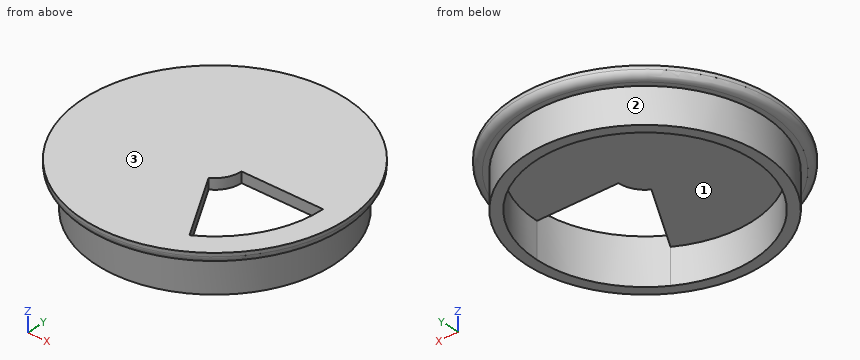
```python
from build123d import *

# Parameters (mm, degrees)
F0_R     = 37
F1_DEPTH = 3
F2_R     = 2
F3_R     = 33.5
F4_DEPTH = 10


with BuildPart() as f1:
    # F0 (on Top) → F1 (new body)
    with BuildSketch(Plane.XY):
        Circle(F0_R)
        with BuildLine():
            ThreePointArc((16.75, -29.0118510268), (-29.0118510268, 16.75), (33.5, 0))
            ThreePointArc((33.5, 0), (29.0118510268, -16.75), (16.75, -29.0118510268))
        make_face(mode=Mode.SUBTRACT)
        with BuildLine():
            Line((7.5, 0), (30.5, 0))
            ThreePointArc((30.5, 0), (-26.4137748154, 15.25), (15.25, -26.4137748154))
            Line((15.25, -26.4137748154), (3.75, -6.4951905284))
            ThreePointArc((3.75, -6.4951905284), (-6.4951905284, 3.75), (7.5, 0))
        make_face()
        with BuildLine():
            Line((30.5, 0), (33.5, 0))
            ThreePointArc((33.5, 0), (-29.0118510268, 16.75), (16.75, -29.0118510268))
            Line((16.75, -29.0118510268), (15.25, -26.4137748154))
            ThreePointArc((15.25, -26.4137748154), (-26.4137748154, 15.25), (30.5, 0))
        make_face()
        with BuildLine():
            ThreePointArc((3.75, -6.4951905284), (6.4951905284, -3.75), (7.5, 0))
            ThreePointArc((7.5, 0), (-6.4951905284, 3.75), (3.75, -6.4951905284))
        make_face()
        with BuildLine():
            ThreePointArc((16.75, -29.0118510268), (29.0118510268, -16.75), (33.5, 0))
            Line((33.5, 0), (30.5, 0))
            ThreePointArc((30.5, 0), (26.4137748154, -15.25), (15.25, -26.4137748154))
            Line((15.25, -26.4137748154), (16.75, -29.0118510268))
        make_face()
    extrude(amount=-F1_DEPTH)

    # F2
    f2_edges = [f1.edges().sort_by_distance(p)[0] for p in [
        (-37, 0, -3),
    ]]
    fillet(f2_edges, radius=F2_R)

    # F3 (on face) → F4 (join)
    with BuildSketch(Plane(origin=(0, 0, -3), x_dir=(1, 0, 0), z_dir=(0, 0, -1))):
        Circle(F3_R)
        with BuildLine():
            ThreePointArc((15.25, 26.4137748154), (26.4137748154, 15.25), (30.5, 0))
            ThreePointArc((30.5, 0), (-26.4137748154, -15.25), (15.25, 26.4137748154))
        make_face(mode=Mode.SUBTRACT)
    extrude(amount=F4_DEPTH)


solid = f1.part
```
Read the model definition and answer for the solid it produces. Units are mm, in the model's axes. Face numbers are marked on the shaded views. Coordinates: 2 decimals unless noted, no trailing zeros. Write each loop counter-clockwise with the first axis right and the second up, starting at its lowest first coordinate (ties: lowest second). Pieces come first, ordered by that corner, then holes. Notation, with made-up numbers: (75.25, -28) -> (112.25, -28) arc R35 cw to (112.25, 11) -> close; hole circle Ø2 at (-13, -18). An arc over 180 degrees is marked (long way). Return JSON: item names as keys, results as strings.
1. Each of these flat-tipped pins is pushed along its axis until it touches: P1, Ø1, axis at x = 13, z = -5.5, coming from the +Y side; P2, Ø6, axis at y = 18.5, z = -2.5, coming from the +X side; P3, Ø1, axis at x = -8.5, y = -15.5, coming from the +Z side; P4, Ø3.5, axis at x = 16, z = -2, coming from the -Y side. Where does it stop, or does it pass through?
Found:
{"P1": "y = 31.08", "P2": "x = 33.46", "P3": "z = 0", "P4": "y = -34.06"}
2. A cutting plane is placed at A-A (x = 0). Determine the outline of the cut face in (y, z).
Found:
{"outline": "(-37, -1) arc R2 ccw to (-35, -3) -> (-33.5, -3) -> (-33.5, -13) -> (-30.5, -13) -> (-30.5, -3) -> (30.5, -3) -> (30.5, -13) -> (33.5, -13) -> (33.5, -3) -> (35, -3) arc R2 ccw to (37, -1) -> (37, 0) -> (-37, 0) -> close"}
3. Determine the mould class of the marked faces 1, 2 and 3 for opening direction Y: pulls with the +Y half, pulls with the -Y half, needs draft (parallel to the pull), parting line crosses it, or undercut.
Found:
{"face 1": "undercut", "face 2": "parting line crosses it", "face 3": "needs draft"}
4. Find the intervals of material crossed by line 1 along Y through (x, z) = (0, -9); line 2 along Z through (x, y) = (-25.5, 8); line 3 along Y through (x, z) = (20.5, -7.5), in increasing order. Write a range as from..to.
Found:
{"line 1": "-33.5..-30.5, 30.5..33.5", "line 2": "-3..0", "line 3": "-26.5..-22.58, 22.58..26.5"}
5. A cutting plane is placed at B-B (z = -10.5). Determine the outline of the cut face in (x, y), and give its area (3 significant figures).
Found:
{"outline": "circle Ø67 at (0, 0); hole circle Ø61 at (0, 0)", "area": "603 mm2"}
